```python
from build123d import *

# Parameters (mm, degrees)
F0_R     = 2.5
F1_DEPTH = 2
F2_R     = 4
F3_DEPTH = 5
F4_R     = 2.5
F5_DEPTH = 7.001


with BuildPart() as f1:
    # F0 (on Top) → F1 (new body)
    with BuildSketch(Plane.XY):
        with BuildLine():
            Line((-1.686594, 34.226591), (-3.492007, 6.637461))
            ThreePointArc((-3.492007, 6.637461), (0, -7.5), (3.492007, 6.637461))
            Line((3.492007, 6.637461), (1.686594, 34.226591))
            ThreePointArc((1.686594, 34.226591), (3.991463, 38.114827), (1.199533, 41.669532))
            Line((1.199533, 41.669532), (0.199573, 56.950255))
            ThreePointArc((0.199573, 56.950255), (0, 57.137195), (-0.199573, 56.950255))
            Line((-0.199573, 56.950255), (-1.199533, 41.669532))
            ThreePointArc((-1.199533, 41.669532), (-3.991463, 38.114827), (-1.686594, 34.226591))
        make_face()
        with Locations((0, 37.853628)):
            Circle(F0_R, mode=Mode.SUBTRACT)
    extrude(amount=F1_DEPTH)

    # F2 (on face) → F3 (join)
    with BuildSketch(Plane.XY.offset(2)):
        Circle(F2_R)
    extrude(amount=F3_DEPTH)

    # F4 (on face) → F5 (cut, through all)
    with BuildSketch(Plane.XY.offset(7)):
        Circle(F4_R)
    extrude(amount=-F5_DEPTH, mode=Mode.SUBTRACT)


solid = f1.part
```
The listing builds one solid part. Answer for the finished solid, in the listing's coordinates (mm). A direction names the side the tool comes from. Round coordinates to 2 decimals unless told otherwise and drop trailing zeros. Loops run counter-clockwise (first coordinate to the right, second up) from the corner with the lowest first, then second, coordinate; pieces in that order, holes last. Notation, with made-up numbers: (-32, 18) - (-18, 18) arc R13 ccw to (-18, 26) - close; hole circle Ø4 at (23.25, 57). An arc over 180 degrees is marked (long way). Return JSON: item names as keys, results as strings. Group by question number.
1. The mould has two halves that part along Y. Classify faces 1 (the flat face through (0, 18, 0)), 2 (the flat face through (0.707, 49.203, 0.986)), 3 (the flat face through (-2.577, 20.625, 0.986)): pulls with the +Y half, pulls with the -Y half, needs draft (parallel to the pull), parting line crosses it, or undercut.
2. The part is cut by section B-B on z = 5.5. Determine the outline of the cut face in (x, y), then the cut area to 3 significant figures.
3. The part is cut by section D-D on y = 50. Determine the outline of the cut face in (x, z).
4. Consider probe 1 along Y at (x, z) = (0, 1.5); probe 2 along Y at (x, z) = (0, 3.75); probe 3 along Z at (x, y) = (-1.75, 29.5). Determine where each line is inside the solid, lowest interval first.
5. The part is cut by section C-C on y = 39.5. Determine the outline of the cut face in (x, z).
6. Which of the six approach directions +Z, -Z, +X, -X, +Y, -Y give full straight-line access (tool end or side, diameter ignored) to faces 4 (the flat face through (0, 15, 2)), 5 (the flat face through (2.6, 20.24, 0.99)), 6 (the flat face through (-0.693, 49.417, 0.986))?
7. The part is cut by section A-A on y = 0. Determine the outline of the cut face in (x, z), then the cut area to 3 significant figures.
8. Each of these flat-tipped pins is pushed along its axis until it touches: P1, Ø1, axis at x = -3, y = 12.5, coming from the +Z side; P2, Ø3, axis at y = 26.5, z = 1, coming from the -X side; P3, Ø4, axis at x = -0.5, z = 6, coming from the +Y side. Where does it stop, or does it pass through?
Resolved:
{
 "1": {"face 1": "needs draft", "face 2": "pulls with the +Y half", "face 3": "undercut"},
 "2": {"outline": "circle Ø8 at (0, 0); hole circle Ø5 at (0, 0)", "area": "30.6 mm²"},
 "3": {"outline": "(-0.65, 0) - (0.65, 0) - (0.65, 2) - (-0.65, 2) - close"},
 "4": {"probe 1": "y = -7.5 to -2.5, 2.5 to 35.35, 40.35 to 57.14", "probe 2": "y = -4 to -2.5, 2.5 to 4", "probe 3": "z = 0 to 2"},
 "5": {"outline": "(-3.65, 0) - (-1.88, 0) - (-1.88, 2) - (-3.65, 2) - close; (1.88, 0) - (3.65, 0) - (3.65, 2) - (1.88, 2) - close"},
 "6": {"face 4": "+Z", "face 5": "+Z, -Z, +X", "face 6": "+Z, -Z, -X, +Y"},
 "7": {"outline": "(-7.5, 0) - (-2.5, 0) - (-2.5, 7) - (-4, 7) - (-4, 2) - (-7.5, 2) - close; (2.5, 0) - (7.5, 0) - (7.5, 2) - (4, 2) - (4, 7) - (2.5, 7) - close", "area": "35.0 mm²"},
 "8": {"P1": "stops at z = 2", "P2": "stops at x = -2.29", "P3": "stops at y = 4"}
}
